The listing builds one solid part. Answer for the finished solid, in the listing's coordinates (mm). A direction names the side the tool comes from. Round coordinates to 2 decimals unless told otherwise and drop trailing zeros. Order: outer loops, then holes, each group sorted by start corner. A loop starts at its lowest first (then second) coordinate and runs counter-clockwise, first axis right, second up. Notation, with made-up numbers: (-10.75, 83.5) -> (36.25, 83.5) arc R19 ccw to (36.25, 120.5) -> close; hole circle Ø1 at (36.25, 37). An arc over 180 degrees is marked (long way). Answer in a Markdown table with one row per item. Add a question column.
```python
from build123d import *

# Parameters (mm, degrees)
SKETCH1_R           = 27
SKETCH1_R_2         = 26
BOSS_EXTRUDE1_DEPTH = 12
BOSS_EXTRUDE2_START = 1
SKETCH2_R           = 27
BOSS_EXTRUDE2_DEPTH = 1
SKETCH3_R           = 25.5
SKETCH3_R_2         = 24.5
BOSS_EXTRUDE3_DEPTH = 0.6
FILLET1_R           = 1
FILLET2_R           = 0.5


with BuildPart() as part:
    # Sketch1 → Boss-Extrude1 (new body)
    with BuildSketch(Plane(origin=(0, 0, 0), x_dir=(1, 0, 0), z_dir=(0, 1, 0))):
        with Locations(Location((0, 0, 0), (0, 0, 270))):
            Circle(SKETCH1_R)
        with Locations(Location((0, 0, 0), (0, 0, 270))):
            Circle(SKETCH1_R_2, mode=Mode.SUBTRACT)
    extrude(amount=BOSS_EXTRUDE1_DEPTH)

    # Sketch2 → Boss-Extrude2 (add)
    with BuildSketch(Plane.XZ.offset(BOSS_EXTRUDE2_START)):
        with Locations(Location((0, 0, 0), (0, 0, 270))):
            Circle(SKETCH2_R)
    extrude(amount=-BOSS_EXTRUDE2_DEPTH)

    # Sketch3 → Boss-Extrude3 (add)
    with BuildSketch(Plane.XZ.offset(1)):
        with Locations(Location((0, 0, 0), (0, 0, 270))):
            Circle(SKETCH3_R)
        with Locations(Location((0, 0, 0), (0, 0, 270))):
            Circle(SKETCH3_R_2, mode=Mode.SUBTRACT)
    extrude(amount=BOSS_EXTRUDE3_DEPTH)

    # Fillet1
    fillet1_edges = [part.edges().sort_by_distance(p)[0] for p in [
        (0, -1, 27),
    ]]
    fillet(fillet1_edges, radius=FILLET1_R - 0.0001)  # a hair under: the kernel refuses the full size

    # Fillet2
    fillet2_edges = [part.edges().sort_by_distance(p)[0] for p in [
        (0, -1.6, 25.5),
        (0, -1.6, 24.5),
    ]]
    fillet(fillet2_edges, radius=FILLET2_R - 0.0001)  # a hair under: the kernel refuses the full size


solid = part.part
```
Item 1: The part is cut by section C-C, the plane y = 9. Give the vertices of the cut face in (x, z).
Item 2: For a pull along Z with two mould halves and no side action, classify faces 3 (the face through (22.1, 12, -14.1)), 4 (the face through (0, -1, 0)) as released by +Z, released by -Z, zero draft, split by the parting line, or undercut.
Item 3: Find the intervals of material crossed by probe 1 along X at (y, z) = (5.5, 0); probe 2 along Y at (x, z) = (2, 10.5); probe 3 along X at (y, z) = (-1.1, 0), in increasing order. Write a range as [from, to].
Item 4: Flat-ended cylindrical pins translate along their axes: P1, Ø2, axis at x = -6, z = -19.5, coming from the +Y side; P2, Ø3, axis at x = 1, z = 20, coming from the -Y side; P3, Ø4, axis at y = 9.5, z = -12.5, coming from the +X side. Find the tip coordinate at first contact, or state that the pin passes through.
Item 5: A tool of negligible diameter and unlimited length cuts with its end or side. For faces 1 (the face through (-15.821, 5.916, -20.633)), 2 (the face through (-17.2, -1, -19.1)), from which of +Z, -Z, +X, -X, +Y, -Y can it reach the whole face along a straight path? Write none if from no direction.
Resolved:
| question | item | result |
|---|---|---|
| 1 | outline | circle Ø54 at (0, 0); hole circle Ø52 at (0, 0) |
| 2 | face 3 | zero draft |
| 2 | face 4 | undercut |
| 3 | probe 1 | [-27, -26], [26, 27] |
| 3 | probe 2 | [-1, 0] |
| 3 | probe 3 | [-25.5, -24.5], [24.5, 25.5] |
| 4 | P1 | y = 0 |
| 4 | P2 | y = -1 |
| 4 | P3 | x = 24.87 |
| 5 | face 1 | +Y |
| 5 | face 2 | -Y |
